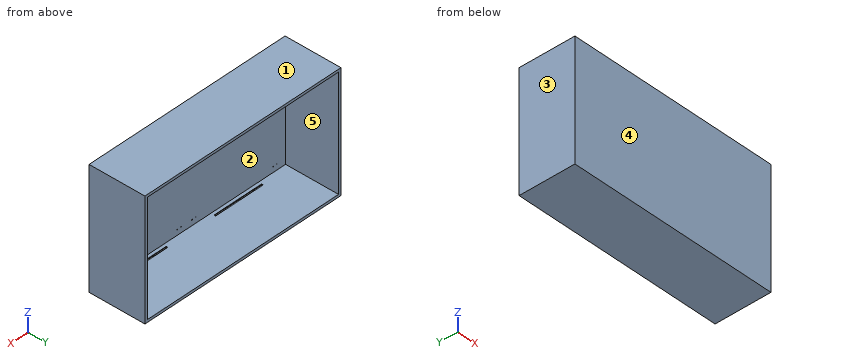
```python
from build123d import *

# Parameters (mm, degrees)
CROQUIS1_W                       = 1320
CROQUIS1_H                       = 740
SALIENTE_EXTRUIR1_DEPTH          = 350
CROQUIS2_W                       = 1288
CROQUIS2_H                       = 708
CORTAR_EXTRUIR1_DEPTH            = 332
TALADRO_DE_MARGEN_PARA_M61_D     = 6
TALADRO_DE_MARGEN_PARA_M61_DEPTH = 1
TALADRO_DE_MARGEN_PARA_M62_D     = 6
TALADRO_DE_MARGEN_PARA_M62_DEPTH = 1
CORTAR_EXTRUIR2_START            = -143
CROQUIS7_W                       = 5
CROQUIS7_H                       = 10.328249786
CORTAR_EXTRUIR2_DEPTH            = 320
CORTAR_EXTRUIR3_START            = -183
CROQUIS8_W                       = 5
CROQUIS8_H                       = 10.328249786
CORTAR_EXTRUIR3_DEPTH            = 320


with BuildPart() as part:
    # Croquis1 → Saliente-Extruir1 (new body)
    with BuildSketch(Plane(origin=(0, 0, 0), x_dir=(1, 0, 0), z_dir=(0, 1, 0))):
        Rectangle(CROQUIS1_W, CROQUIS1_H)
    extrude(amount=SALIENTE_EXTRUIR1_DEPTH)

    # Croquis2 → Cortar-Extruir1 (cut)
    with BuildSketch(Plane(origin=(0, 350, 0), x_dir=(1, 0, 0), z_dir=(0, 1, 0))):
        Rectangle(CROQUIS2_W, CROQUIS2_H)
    extrude(amount=-CORTAR_EXTRUIR1_DEPTH, mode=Mode.SUBTRACT)

    # Taladro de margen para M61
    with Locations(Plane(origin=(275.040116616, 18, -214.423302292), x_dir=(1, 0, 0), z_dir=(0, 1, 0))):
        with Locations((-831.164543187, -520.352285028), (-831.164543187, -546.055205699), (-855.664607514, -546.055205699), (-855.664607514, -520.352285028)):
            Hole(TALADRO_DE_MARGEN_PARA_M61_D / 2, depth=TALADRO_DE_MARGEN_PARA_M61_DEPTH)

    # Taladro de margen para M62
    with Locations(Plane(origin=(275.040116616, 18, -214.423302292), x_dir=(1, 0, 0), z_dir=(0, 1, 0))):
        with Locations((-859.800116616, 105.076697708), (-834.300547142, 105.075612323), (-314.039673698, 105.075612323), (-288.540104225, 105.075612323), (-214.748048522, 105.075612323), (-188.969749284, 105.075612323), (326.914692955, 105.075612323), (352.414262429, 105.075612323), (323.921080143, -520.352285028), (348.42114447, -520.352285028), (348.42114447, -546.055205699), (323.921080143, -546.055205699), (-185.793163735, -520.352285028), (-185.793163735, -546.055205699), (-214.649068849, -547.297061638), (-210.293228062, -520.352285028), (-292.457959943, -520.352285028), (-292.457959943, -546.055205699), (-316.95802427, -546.055205699), (-316.95802427, -520.352285028)):
            Hole(TALADRO_DE_MARGEN_PARA_M62_D / 2, depth=TALADRO_DE_MARGEN_PARA_M62_DEPTH)

    # Croquis7 → Cortar-Extruir2 (cut)
    with BuildSketch(Plane(origin=(644, 0, -214.423302292), x_dir=(0, 0, -1), z_dir=(1, 0, 0)).offset(CORTAR_EXTRUIR2_START)):
        with Locations((142.076697708, 42.95033831)):
            Rectangle(CROQUIS7_W, CROQUIS7_H)
    extrude(amount=-CORTAR_EXTRUIR2_DEPTH, mode=Mode.SUBTRACT)

    # Croquis8 → Cortar-Extruir3 (cut)
    with BuildSketch(Plane(origin=(-644, 0, -214.423302292), x_dir=(0, 0, 1), z_dir=(-1, 0, 0)).offset(CORTAR_EXTRUIR3_START)):
        with Locations((-142.076697708, 42.95033831)):
            Rectangle(CROQUIS8_W, CROQUIS8_H)
    extrude(amount=-CORTAR_EXTRUIR3_DEPTH, mode=Mode.SUBTRACT)


solid = part.part
```
Geometry: final body of the model. Coordinates: model frame, mm. Face numbers are marked on the shaded views. A direction names the side the tool comes from. Round coordinates to 2 decimals unless told otherwise and drop trailing zeros. Write each loop counter-clockwise with the first axis right and the second up, starting at its lowest first coordinate (ties: lowest second). Pieces come first, ordered by that corner, then holes.
Item 1: Section query A-A (y = 281). Return loops of the section in (x, z).
Item 2: Pin query (flat end, axial travel): P1, Ø7, axis at x = -556.12, z = 305.93, coming from the +Y side; P2, Ø1.8, axis at x = -41, z = 331, coming from the +Y side. Return the tip coordinate at first contact, or that it passes through.
Item 3: Mould query, pull axis Z, two halves, no side actions, for the marked faces 1, 2 and 3. Classes: +Z half, -Z half, draft (parallel to the pull), parting line (faces both ways), or undercut.
Item 4: Section query C-C (x = 569.5). Return loops of the section in (y, z), plus the area to 3 significant figures.
Item 5: Material intervals for L1, parallel to Z at x = 490.5, y = 57; L2, parallel to X at y = 335.5, z = 118.5; L3, parallel to Z at x = 368.5, y = 39, sorted ascending.
Item 6: Set-up query: the marked faces 4 and 5. Return all of +Z, -Z, +X, -X, +Y, -Y with unobstructed straight access to the full face (end or side cutting, diameter ignored); none if empty.
Item 7: Section query B-B (z = 118.5). Return loops of the section in (x, y), plus the area to 3 significant figures.
Completed:
1. outline: (-660, -370) - (660, -370) - (660, 370) - (-660, 370) - close; hole (-644, -354) - (644, -354) - (644, 354) - (-644, 354) - close
2. P1: stops at y = 18
2. P2: stops at y = 17
3. face 1: +Z half
3. face 2: undercut
3. face 3: draft
4. outline: (0, -370) - (350, -370) - (350, -354) - (18, -354) - (18, 354) - (350, 354) - (350, 370) - (0, 370) - close
4. area: 23,900 mm2
5. L1: z = -370 to -354, 354 to 370
5. L2: x = -660 to -644, 644 to 660
5. L3: z = -370 to -359, 354 to 370
6. face 4: +Z, -Z, +X, -X, -Y
6. face 5: +Y
7. outline: (-660, 0) - (660, 0) - (660, 350) - (644, 350) - (644, 18) - (-644, 18) - (-644, 350) - (-660, 350) - close
7. area: 34,400 mm2
